Input: dimensioned drawing with shaded views. Units: mm. Origin: part minimum x, y, z. Round coordinates to 2 decimals unless told otherwise and drop trailing zeros. Order: outer loops, then holes, each group sorted by start corner. A loop starts at its lowest first (then second) coordinate and runs counter-clockwise, first axis right, second up. Notation, with made-up numbers: (-36, 24) - (-1, 24) arc R25 cw to (-1, 53) - close; hole circle Ø3 at (50, -18.75). An arc over 180 degrees is marked (long way). Put each result on its own line as item: value. Start each with the question number.
(1) Pull-direction query (Y, two-part tool) for the marked faces 1, 2, 3 and 4; classes: released by +Y, released by -Y, zero draft, split by the parting line, or undercut.
(2) Material intervals for L1, parallel to Y at x = 10, z = 2.5; L2, parallel to X at y = 12.5, z = 8; L3, parallel to X at y = 12, z = 5, sorted ascending. Write a range as [from, to].
(3) Section C-C (y = 25). Output: boundary loops of the cut face in (x, z).
(4) Section A-A (z = 89.5). Output: boundary loops of the cut face in (x, y).
(5) Pin query (flat end, axial travel): P1, Ø2, axis at x = 17.5, y = 35.5, coming from the +Z side; P2, Ø6.5, axis at x = 10, y = 12.5, coming from the -Z side. Return the tip coordinate at first contact, or that it passes through.
(6) Section D-D (y = 31). Output: boundary loops of the cut face in (x, z).
(7) Section B-B (x = 16.25). Output: boundary loops of the cut face in (y, z).
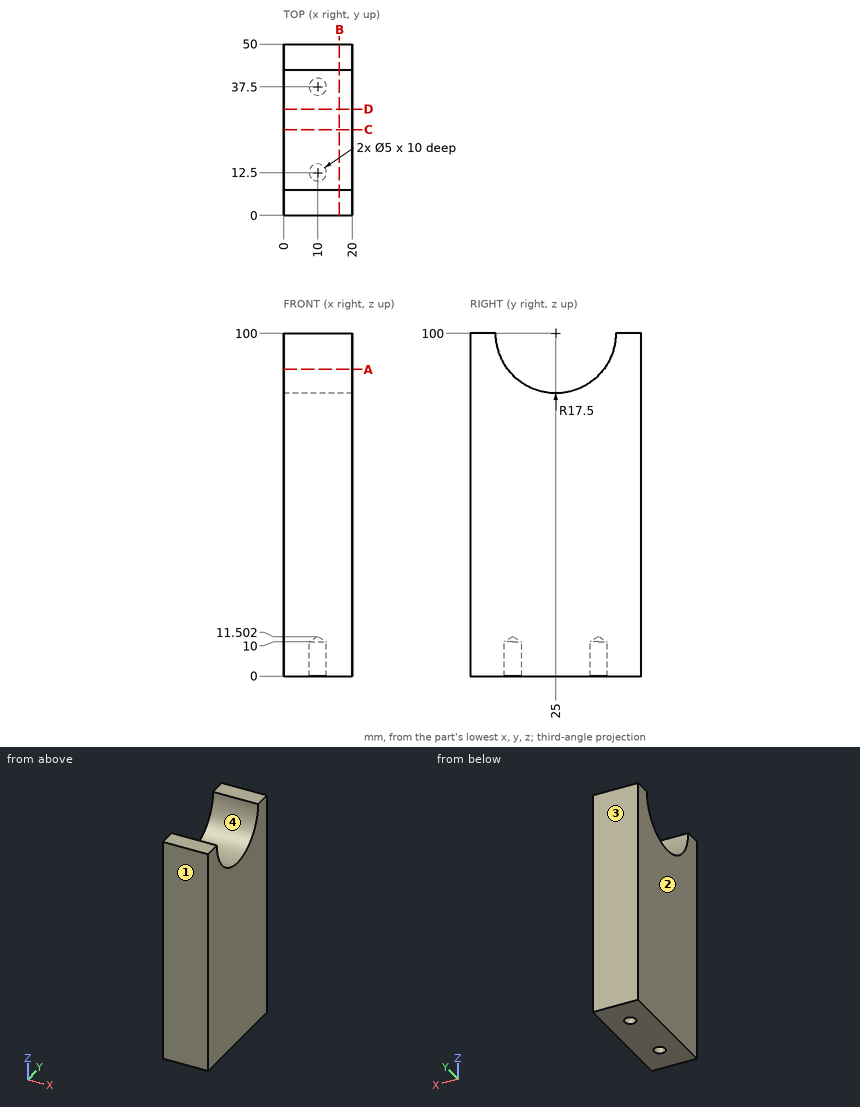
Checks:
1. face 1: released by -Y
1. face 2: zero draft
1. face 3: released by +Y
1. face 4: undercut
2. L1: y = [0, 10], [15, 35], [40, 50]
2. L2: x = [0, 7.5], [12.5, 20]
2. L3: x = [0, 7.55], [12.45, 20]
3. outline: (0, 0) - (20, 0) - (20, 82.5) - (0, 82.5) - close
4. outline: (0, 0) - (20, 0) - (20, 11) - (0, 11) - close; (0, 39) - (20, 39) - (20, 50) - (0, 50) - close
5. P1: stops at z = 86.81
5. P2: stops at z = 0
6. outline: (0, 0) - (20, 0) - (20, 83.56) - (0, 83.56) - close
7. outline: (0, 0) - (50, 0) - (50, 100) - (42.5, 100) arc R17.5 cw to (7.5, 100) - (0, 100) - close
